Can you work these out from the model? Positions are in its coordinate system, mm. A direction names the side the tool comes from. Give positions to 0.01 mm unless a question says otherwise; leave off trailing zeros. Write each question's results on one line, items separated by ' | '.
from build123d import *

# Parameters (mm, degrees)
CYLINDER297_R               = 3
CYLINDER297_DEPTH           = 3
CYLINDER297_PLACEMENT_ANGLE = 45
CYLINDER296_R               = 3
CYLINDER296_DEPTH           = 3
CYLINDER293_R               = 3
CYLINDER293_DEPTH           = 3
CYLINDER293_PLACEMENT_ANGLE = 135
CYLINDER298_R               = 3
CYLINDER298_DEPTH           = 3
CYLINDER292_R               = 3
CYLINDER292_DEPTH           = 3
CYLINDER292_PLACEMENT_ANGLE = 225
CYLINDER295_R               = 3
CYLINDER295_DEPTH           = 3
CYLINDER299_R               = 3
CYLINDER299_DEPTH           = 3
CYLINDER299_PLACEMENT_ANGLE = 45
CYLINDER294_R               = 3
CYLINDER294_DEPTH           = 3
COMPOUND237_PLACEMENT_ANGLE = 22.5
CYLINDER288_R               = 1.5
CYLINDER288_DEPTH           = 20
CYLINDER288_PLACEMENT_ANGLE = 45
CYLINDER284_R               = 1.5
CYLINDER284_DEPTH           = 20
CYLINDER285_R               = 1.5
CYLINDER285_DEPTH           = 20
CYLINDER285_PLACEMENT_ANGLE = 135
CYLINDER291_R               = 1.5
CYLINDER291_DEPTH           = 20
CYLINDER289_R               = 1.5
CYLINDER289_DEPTH           = 20
CYLINDER289_PLACEMENT_ANGLE = 225
CYLINDER287_R               = 1.5
CYLINDER287_DEPTH           = 20
CYLINDER290_R               = 1.5
CYLINDER290_DEPTH           = 20
CYLINDER290_PLACEMENT_ANGLE = 45
CYLINDER286_R               = 1.5
CYLINDER286_DEPTH           = 20
COMPOUND236_PLACEMENT_ANGLE = 22.5
CYLINDER280_R               = 1.5
CYLINDER280_DEPTH           = 16
CYLINDER280_PLACEMENT_ANGLE = 67.5
CYLINDER282_R               = 1.5
CYLINDER282_DEPTH           = 16
CYLINDER282_PLACEMENT_ANGLE = 22.5
CYLINDER283_R               = 1.5
CYLINDER283_DEPTH           = 16
CYLINDER283_PLACEMENT_ANGLE = 112.5
CYLINDER281_R               = 1.5
CYLINDER281_DEPTH           = 16
CYLINDER281_PLACEMENT_ANGLE = 202.5
TUBE029_R                   = 52
TUBE029_R_2                 = 12
TUBE029_DEPTH               = 5
CHAMFER003_SIZE             = 1


with BuildPart() as obj1:
    # Cylinder297 → Cylinder297 (new body)
    with BuildSketch(Plane.XY):
        Circle(CYLINDER297_R)
    extrude(amount=CYLINDER297_DEPTH)


with BuildPart() as obj1_1:
    # Cylinder297 placement: moved
    add(obj1.part.moved(Location((-31.819805, 31.819805, -18))).rotate(Axis((-31.819805, 31.819805, -18), (0, 0, 1)), CYLINDER297_PLACEMENT_ANGLE))


with BuildPart() as obj2:
    # Cylinder296 → Cylinder296 (new body)
    with BuildSketch(Plane(origin=(-45, 0, -18), x_dir=(0, 1, 0), z_dir=(0, 0, 1))):
        Circle(CYLINDER296_R)
    extrude(amount=CYLINDER296_DEPTH)


with BuildPart() as obj3:
    # Cylinder293 → Cylinder293 (new body)
    with BuildSketch(Plane.XY):
        Circle(CYLINDER293_R)
    extrude(amount=CYLINDER293_DEPTH)


with BuildPart() as obj3_1:
    # Cylinder293 placement: moved
    add(obj3.part.moved(Location((-31.819805, -31.819805, -18))).rotate(Axis((-31.819805, -31.819805, -18), (0, 0, 1)), CYLINDER293_PLACEMENT_ANGLE))


with BuildPart() as obj4:
    # Cylinder298 → Cylinder298 (new body)
    with BuildSketch(Plane(origin=(0, -45, -18), x_dir=(-1, 0, 0), z_dir=(0, 0, 1))):
        Circle(CYLINDER298_R)
    extrude(amount=CYLINDER298_DEPTH)


with BuildPart() as obj5:
    # Cylinder292 → Cylinder292 (new body)
    with BuildSketch(Plane.XY):
        Circle(CYLINDER292_R)
    extrude(amount=CYLINDER292_DEPTH)


with BuildPart() as obj5_1:
    # Cylinder292 placement: moved
    add(obj5.part.moved(Location((31.819805, -31.819805, -18))).rotate(Axis((31.819805, -31.819805, -18), (0, 0, 1)), CYLINDER292_PLACEMENT_ANGLE))


with BuildPart() as obj6:
    # Cylinder295 → Cylinder295 (new body)
    with BuildSketch(Plane(origin=(45, 0, -18), x_dir=(0, -1, 0), z_dir=(0, 0, 1))):
        Circle(CYLINDER295_R)
    extrude(amount=CYLINDER295_DEPTH)


with BuildPart() as obj7:
    # Cylinder299 → Cylinder299 (new body)
    with BuildSketch(Plane.XY):
        Circle(CYLINDER299_R)
    extrude(amount=CYLINDER299_DEPTH)


with BuildPart() as obj7_1:
    # Cylinder299 placement: moved
    add(obj7.part.moved(Location((31.819805, 31.819805, -18))).rotate(Axis((31.819805, 31.819805, -18), (0, 0, -1)), CYLINDER299_PLACEMENT_ANGLE))


with BuildPart() as compound237:
    # Cylinder294 → Cylinder294 (new body)
    with BuildSketch(Plane(origin=(0, 45, -18), x_dir=(1, 0, 0), z_dir=(0, 0, 1))):
        Circle(CYLINDER294_R)
    extrude(amount=CYLINDER294_DEPTH)

    # Compound237: union obj1, obj2, obj3, obj4, obj5, obj6, obj7
    add(obj1_1.part)
    add(obj2.part)
    add(obj3_1.part)
    add(obj4.part)
    add(obj5_1.part)
    add(obj6.part)
    add(obj7_1.part)


with BuildPart() as compound237_1:
    # Compound237 placement: moved
    add(compound237.part.moved(Location((0, 0, -82))).rotate(Axis((0, 0, -82), (0, 0, 1)), COMPOUND237_PLACEMENT_ANGLE))


with BuildPart() as obj8:
    # Cylinder288 → Cylinder288 (new body)
    with BuildSketch(Plane.XY):
        Circle(CYLINDER288_R)
    extrude(amount=CYLINDER288_DEPTH)


with BuildPart() as obj8_1:
    # Cylinder288 placement: moved
    add(obj8.part.moved(Location((-31.819805, 31.819805, -18))).rotate(Axis((-31.819805, 31.819805, -18), (0, 0, 1)), CYLINDER288_PLACEMENT_ANGLE))


with BuildPart() as obj9:
    # Cylinder284 → Cylinder284 (new body)
    with BuildSketch(Plane(origin=(-45, 0, -18), x_dir=(0, 1, 0), z_dir=(0, 0, 1))):
        Circle(CYLINDER284_R)
    extrude(amount=CYLINDER284_DEPTH)


with BuildPart() as obj10:
    # Cylinder285 → Cylinder285 (new body)
    with BuildSketch(Plane.XY):
        Circle(CYLINDER285_R)
    extrude(amount=CYLINDER285_DEPTH)


with BuildPart() as obj10_1:
    # Cylinder285 placement: moved
    add(obj10.part.moved(Location((-31.819805, -31.819805, -18))).rotate(Axis((-31.819805, -31.819805, -18), (0, 0, 1)), CYLINDER285_PLACEMENT_ANGLE))


with BuildPart() as obj11:
    # Cylinder291 → Cylinder291 (new body)
    with BuildSketch(Plane(origin=(0, -45, -18), x_dir=(-1, 0, 0), z_dir=(0, 0, 1))):
        Circle(CYLINDER291_R)
    extrude(amount=CYLINDER291_DEPTH)


with BuildPart() as obj12:
    # Cylinder289 → Cylinder289 (new body)
    with BuildSketch(Plane.XY):
        Circle(CYLINDER289_R)
    extrude(amount=CYLINDER289_DEPTH)


with BuildPart() as obj12_1:
    # Cylinder289 placement: moved
    add(obj12.part.moved(Location((31.819805, -31.819805, -18))).rotate(Axis((31.819805, -31.819805, -18), (0, 0, 1)), CYLINDER289_PLACEMENT_ANGLE))


with BuildPart() as obj13:
    # Cylinder287 → Cylinder287 (new body)
    with BuildSketch(Plane(origin=(45, 0, -18), x_dir=(0, -1, 0), z_dir=(0, 0, 1))):
        Circle(CYLINDER287_R)
    extrude(amount=CYLINDER287_DEPTH)


with BuildPart() as obj14:
    # Cylinder290 → Cylinder290 (new body)
    with BuildSketch(Plane.XY):
        Circle(CYLINDER290_R)
    extrude(amount=CYLINDER290_DEPTH)


with BuildPart() as obj14_1:
    # Cylinder290 placement: moved
    add(obj14.part.moved(Location((31.819805, 31.819805, -18))).rotate(Axis((31.819805, 31.819805, -18), (0, 0, -1)), CYLINDER290_PLACEMENT_ANGLE))


with BuildPart() as compound236:
    # Cylinder286 → Cylinder286 (new body)
    with BuildSketch(Plane(origin=(0, 45, -18), x_dir=(1, 0, 0), z_dir=(0, 0, 1))):
        Circle(CYLINDER286_R)
    extrude(amount=CYLINDER286_DEPTH)

    # Compound236: union obj8, obj9, obj10, obj11, obj12, obj13, obj14
    add(obj8_1.part)
    add(obj9.part)
    add(obj10_1.part)
    add(obj11.part)
    add(obj12_1.part)
    add(obj13.part)
    add(obj14_1.part)


with BuildPart() as compound236_1:
    # Compound236 placement: moved
    add(compound236.part.moved(Location((0, 0, -87))).rotate(Axis((0, 0, -87), (0, 0, 1)), COMPOUND236_PLACEMENT_ANGLE))


with BuildPart() as obj15:
    # Cylinder280 → Cylinder280 (new body)
    with BuildSketch(Plane.XY):
        Circle(CYLINDER280_R)
    extrude(amount=CYLINDER280_DEPTH)


with BuildPart() as obj15_1:
    # Cylinder280 placement: moved
    add(obj15.part.moved(Location((0, 16, 2))).rotate(Axis((0, 16, 2), (0, 0, -1)), CYLINDER280_PLACEMENT_ANGLE))


with BuildPart() as obj16:
    # Cylinder282 → Cylinder282 (new body)
    with BuildSketch(Plane.XY):
        Circle(CYLINDER282_R)
    extrude(amount=CYLINDER282_DEPTH)


with BuildPart() as obj16_1:
    # Cylinder282 placement: moved
    add(obj16.part.moved(Location((-16, 0, 2))).rotate(Axis((-16, 0, 2), (0, 0, 1)), CYLINDER282_PLACEMENT_ANGLE))


with BuildPart() as obj17:
    # Cylinder283 → Cylinder283 (new body)
    with BuildSketch(Plane.XY):
        Circle(CYLINDER283_R)
    extrude(amount=CYLINDER283_DEPTH)


with BuildPart() as obj17_1:
    # Cylinder283 placement: moved
    add(obj17.part.moved(Location((0, -16, 2))).rotate(Axis((0, -16, 2), (0, 0, 1)), CYLINDER283_PLACEMENT_ANGLE))


with BuildPart() as compound235:
    # Cylinder281 → Cylinder281 (new body)
    with BuildSketch(Plane.XY):
        Circle(CYLINDER281_R)
    extrude(amount=CYLINDER281_DEPTH)


with BuildPart() as compound235_1:
    # Cylinder281 placement: moved
    add(compound235.part.moved(Location((16, 0, 2))).rotate(Axis((16, 0, 2), (0, 0, 1)), CYLINDER281_PLACEMENT_ANGLE))

    # Compound235: union obj15, obj16, obj17
    add(obj15_1.part)
    add(obj16_1.part)
    add(obj17_1.part)


with BuildPart() as compound235_2:
    # Compound235 placement: moved
    add(compound235_1.part.moved(Location((0, 0, -117))))


with BuildPart() as chamfer003:
    # Tube029 → Tube029 (new body)
    with BuildSketch(Plane.XY.offset(-100)):
        Circle(TUBE029_R)
        Circle(TUBE029_R_2, mode=Mode.SUBTRACT)
    extrude(amount=TUBE029_DEPTH)

    # Cut125: cut Compound235
    add(compound235_2.part, mode=Mode.SUBTRACT)

    # Cut127: cut Compound236
    add(compound236_1.part, mode=Mode.SUBTRACT)

    # Cut128: cut Compound237
    add(compound237_1.part, mode=Mode.SUBTRACT)

    # Chamfer003
    chamfer003_edges = [chamfer003.edges().sort_by_distance(p)[0] for p in [
        (-52, 0, -100),
    ]]
    chamfer(chamfer003_edges, length=CHAMFER003_SIZE)


solid = chamfer003.part
Item 1: Thinking about a two-plate mould opening in Y: for faces 1 (the face through (-16, 0, -99)), 2 (the face through (-41.265, -31.641, -97.028)), which applies, +Y half, -Y half, draft (parallel to the pull), parting line (faces both ways), or undercut?
Geometry says:
face 1: undercut | face 2: parting line
Item 2: For faces 3 (the face through (-18, 40, -97)), 4 (the face through (16.961, -40.097, -96.014)), which set-ups out of +Z, -Z, +X, -X, +Y, -Y let a thin tool reach every point of the face, with its end or its side?
Geometry says:
face 3: -Z | face 4: +Z, -Z
Item 3: If I drill on line 1 (Y direction, x = -16, z = -99.5); line 2 (Y direction, x = 42, z = -99); line 3 (Y direction, x = -15, z = -97.1), over which ranges is the centre line in solid material (lowest first)? Write a range as from..to.
Geometry says:
line 1: y = -48.95..-44.31, -38.83..-1.5, 1.5..38.83, 44.31..48.95 | line 2: y = -30.66..-20.19, -14.25..14.25, 20.19..30.66 | line 3: y = -49.79..-43.59, -39.56..39.56, 43.59..49.79
Item 4: I want a section at A-A, the plane z = -97.8. Give the number of separate pieces and of enclosed holes in the cut face, and give its area (3 significant figures).
Geometry says:
separate pieces: 1 | enclosed holes: 9 | area: 7,820 mm2
Item 5: I'm going to push flat-ended pins straight in: pin 1 (3 mm diameter, centred on y = -2, z = -96, fed in from -X); pin 2 (1.5 mm diameter, centred on x = -29.5, z = -96, fed in from +Y); pin 3 (1.5 mm diameter, centred on x = 40.5, z = -96.5, fed in from +Y). Where does each tip first touch, or does it pass through?
Geometry says:
pin 1: stops at x = -52 | pin 2: stops at y = 43.33 | pin 3: stops at y = 33.53
